from build123d import *

# Parameters (mm, degrees)
ESQUISSE1_W             = 8.5
ESQUISSE1_H             = 72
ESQUISSE1_R             = 2.1
BOSS_EXTRU_1_DEPTH      = 17.5
ENL_V_START             = -3
ENL_V_MAT_EXTRU_4_DEPTH = 3.5
ESQUISSE7_R             = 2.1
BOSS_EXTRU_3_DEPTH      = 8
ESQUISSE3_W             = 8.5
ESQUISSE3_H             = 4
ENL_V_MAT_EXTRU_3_DEPTH = 19
BOSS_EXTRU_2_START      = -7
BOSS_EXTRU_2_DEPTH      = 12
ESQUISSE8_W             = 8.5
ESQUISSE8_H             = 7
BOSS_EXTRU_4_DEPTH      = 4
ESQUISSE9_R             = 1.6
ENL_V_MAT_EXTRU_5_DEPTH = 5
ENL_V_START_2           = -4
ESQUISSE10_R            = 1.6
ENL_V_MAT_EXTRU_6_DEPTH = 2.6
ESQUISSE11_R            = 1.6
ENL_V_MAT_EXTRU_7_DEPTH = 1.6
ESQUISSE14_W            = 2.5
ESQUISSE14_H            = 10
ENL_V_MAT_EXTRU_9_DEPTH = 17.6
CHANFREIN1_SIZE         = 0.5


with BuildPart() as part:
    # Esquisse1 → Boss.-Extru.1 (new body)
    with BuildSketch(Plane.XY):
        with Locations((4.25, 36)):
            Rectangle(ESQUISSE1_W, ESQUISSE1_H)
        with Locations((4, 20.5)):
            Circle(ESQUISSE1_R, mode=Mode.SUBTRACT)
        with Locations((4, 51.5)):
            Circle(ESQUISSE1_R, mode=Mode.SUBTRACT)
    extrude(amount=BOSS_EXTRU_1_DEPTH)

    # Esquisse6 → Enlèv. mat.-Extru.4 (cut)
    with BuildSketch(Plane.XY.offset(17.5).offset(ENL_V_START)):
        Polygon((7.6, 22.578460969), (4, 24.656921938), (0.4, 22.578460969), (0.4, 18.421539031), (4, 16.343078062), (7.6, 18.421539031), align=None)
        Polygon((8.5, 24.656921938), (4, 24.656921938), (7.6, 22.578460969), (7.6, 18.421539031), (4, 16.343078062), (8.5, 16.343078062), align=None)
    enl_v_mat_extru_4 = extrude(amount=-ENL_V_MAT_EXTRU_4_DEPTH, mode=Mode.SUBTRACT)

    # Esquisse7 → Boss.-Extru.3 (add)
    with BuildSketch(Plane(origin=(0, 0, 0), x_dir=(-1, 0, 0), z_dir=(0, 0, -1))):
        with Locations((-4, 20.5)):
            Circle(ESQUISSE7_R)
    boss_extru_3 = extrude(amount=-BOSS_EXTRU_3_DEPTH)

    # Esquisse3 → Enlèv. mat.-Extru.3 (cut)
    with BuildSketch(Plane(origin=(0, 0, 0), x_dir=(-1, 0, 0), z_dir=(0, -1, 0))):
        with Locations((-4.25, -2)):
            Rectangle(ESQUISSE3_W, ESQUISSE3_H)
    enl_v_mat_extru_3 = extrude(amount=-ENL_V_MAT_EXTRU_3_DEPTH, mode=Mode.SUBTRACT)

    # Esquisse5 → Boss.-Extru.2 (add)
    with BuildSketch(Plane.XZ.offset(BOSS_EXTRU_2_START)):
        with BuildLine():
            ThreePointArc((4.662966643, 2.165487935), (4.682946936, 2.27184931), (4.714353535, 2.375413685))
            ThreePointArc((4.714353535, 2.375413685), (5.229781903, 2.78475984), (5.773646598, 2.414028307))
            ThreePointArc((5.773646598, 2.414028307), (5.814751932, 2.291920009), (5.839789089, 2.165534781))
            ThreePointArc((5.839789089, 2.165534781), (5.889607538, 2.072347427), (5.988503907, 2.035128225))
            Line((5.988503907, 2.035128225), (6.514258005, 2.035128225))
            ThreePointArc((6.514258005, 2.035128225), (6.613136609, 2.072331852), (6.662966643, 2.165487935))
            ThreePointArc((6.662966643, 2.165487935), (6.682946936, 2.27184931), (6.714353535, 2.375413685))
            ThreePointArc((6.714353535, 2.375413685), (7.229781903, 2.78475984), (7.773646598, 2.414028307))
            ThreePointArc((7.773646598, 2.414028307), (7.814751932, 2.291920009), (7.839789089, 2.165534781))
            ThreePointArc((7.839789089, 2.165534781), (7.889607538, 2.072347427), (7.988503907, 2.035128225))
            Line((7.988503907, 2.035128225), (8.5, 2.035128225))
            Line((8.5, 2.035128225), (8.5, 4))
            Line((8.5, 4), (0, 4))
            Line((0, 4), (0, 2.035128225))
            Line((0, 2.035128225), (0.514258005, 2.035128225))
            ThreePointArc((0.514258005, 2.035128225), (0.61313661, 2.072331853), (0.662966644, 2.165487937))
            ThreePointArc((0.662966644, 2.165487937), (0.682946936, 2.271849312), (0.714353535, 2.375413685))
            ThreePointArc((0.714353535, 2.375413685), (1.229781903, 2.78475984), (1.773646598, 2.414028307))
            ThreePointArc((1.773646598, 2.414028307), (1.814751932, 2.291920009), (1.839789089, 2.165534781))
            ThreePointArc((1.839789089, 2.165534781), (1.889607538, 2.072347427), (1.988503907, 2.035128225))
            Line((1.988503907, 2.035128225), (2.514258006, 2.035128225))
            ThreePointArc((2.514258006, 2.035128225), (2.613136611, 2.072331854), (2.662966644, 2.16548794))
            ThreePointArc((2.662966644, 2.16548794), (2.682946936, 2.271849313), (2.714353535, 2.375413685))
            ThreePointArc((2.714353535, 2.375413685), (3.229781903, 2.78475984), (3.773646598, 2.414028307))
            ThreePointArc((3.773646598, 2.414028307), (3.814751932, 2.291920009), (3.839789089, 2.165534781))
            ThreePointArc((3.839789089, 2.165534781), (3.889607538, 2.072347427), (3.988503907, 2.035128225))
            Line((3.988503907, 2.035128225), (4.514258005, 2.035128225))
            ThreePointArc((4.514258005, 2.035128225), (4.613136609, 2.072331852), (4.662966643, 2.165487935))
        make_face()
    boss_extru_2 = extrude(amount=-BOSS_EXTRU_2_DEPTH)

    # Esquisse8 → Boss.-Extru.4 (add)
    with BuildSketch(Plane(origin=(0, 0, 4), x_dir=(-1, 0, 0), z_dir=(0, 0, -1))):
        with Locations((-4.25, 3.5)):
            Rectangle(ESQUISSE8_W, ESQUISSE8_H)
    boss_extru_4 = extrude(amount=BOSS_EXTRU_4_DEPTH)

    # Esquisse9 → Enlèv. mat.-Extru.5 (cut)
    with BuildSketch(Plane(origin=(0, 0, 0), x_dir=(-1, 0, 0), z_dir=(0, 0, -1))):
        with Locations((-4.25, 3.75)):
            Circle(ESQUISSE9_R)
        with Locations((-4.25, 22.25)):
            Circle(ESQUISSE9_R)
    enl_v_mat_extru_5 = extrude(amount=-ENL_V_MAT_EXTRU_5_DEPTH, mode=Mode.SUBTRACT)

    # Esquisse10 → Enlèv. mat.-Extru.6 (cut)
    # profile 1 of 4: a face of its own
    with BuildSketch(Plane(origin=(0, 0, 0), x_dir=(-1, 0, 0), z_dir=(0, 0, -1)).offset(ENL_V_START_2)):
        Polygon((-2.604551733, 25.1), (-5.895448267, 25.1), (-7.540896534, 22.25), (-5.895448267, 19.4), (-2.604551733, 19.4), (-0.959103466, 22.25), align=None)
        with Locations((-4.25, 22.25)):
            Circle(ESQUISSE10_R, mode=Mode.SUBTRACT)
    # profile 2 of 4: a face of its own
    with BuildSketch(Plane(origin=(0, 0, 0), x_dir=(-1, 0, 0), z_dir=(0, 0, -1)).offset(ENL_V_START_2)):
        Polygon((-2.604551733, 6.6), (-5.895448267, 6.6), (-7.540896534, 3.75), (-5.895448267, 0.9), (-2.604551733, 0.9), (-0.959103466, 3.75), align=None)
    # profile 3 of 4: a face of its own
    with BuildSketch(Plane(origin=(0, 0, 0), x_dir=(-1, 0, 0), z_dir=(0, 0, -1)).offset(ENL_V_START_2)):
        Polygon((-8.5, 6.6), (-5.895448267, 6.6), (-7.540896534, 3.75), (-5.895448267, 0.9), (-8.5, 0.9), align=None)
    # profile 4 of 4: a face of its own
    with BuildSketch(Plane(origin=(0, 0, 0), x_dir=(-1, 0, 0), z_dir=(0, 0, -1)).offset(ENL_V_START_2)):
        Polygon((-7.540896534, 22.25), (-5.895448267, 25.1), (-8.5, 25.1), (-8.5, 19.4), (-5.895448267, 19.4), align=None)
    enl_v_mat_extru_6 = extrude(amount=-ENL_V_MAT_EXTRU_6_DEPTH, mode=Mode.SUBTRACT)

    # Esquisse11 → Enlèv. mat.-Extru.7 (cut)
    with BuildSketch(Plane(origin=(0, 0, 5), x_dir=(-1, 0, 0), z_dir=(0, 0, -1))):
        with Locations((-4.25, 22.25)):
            Circle(ESQUISSE11_R)
    enl_v_mat_extru_7 = extrude(amount=-ENL_V_MAT_EXTRU_7_DEPTH, mode=Mode.SUBTRACT)

    # Esquisse14 → Enlèv. mat.-Extru.9 (cut)
    with BuildSketch(Plane(origin=(8.5, 0, 0), x_dir=(0, 0, -1), z_dir=(1, 0, 0))):
        with Locations((-6.75, 13)):
            Rectangle(ESQUISSE14_W, ESQUISSE14_H)
    enl_v_mat_extru_9 = extrude(amount=-ENL_V_MAT_EXTRU_9_DEPTH, mode=Mode.SUBTRACT)

    # Symétrie14: Enlèv. mat.-Extru.4, Boss.-Extru.3, Enlèv. mat.-Extru.3, Boss.-Extru.2, Boss.-Extru.4, Enlèv. mat.-Extru.5, Enlèv. mat.-Extru.6, Enlèv. mat.-Extru.7, Enlèv. mat.-Extru.9 across plane
    add(enl_v_mat_extru_4.mirror(Plane(origin=(0, 36, 0), x_dir=(0, 0, 1), z_dir=(0, -1, 0))), mode=Mode.SUBTRACT)
    add(boss_extru_3.mirror(Plane(origin=(0, 36, 0), x_dir=(0, 0, 1), z_dir=(0, -1, 0))))
    add(enl_v_mat_extru_3.mirror(Plane(origin=(0, 36, 0), x_dir=(0, 0, 1), z_dir=(0, -1, 0))), mode=Mode.SUBTRACT)
    add(boss_extru_2.mirror(Plane(origin=(0, 36, 0), x_dir=(0, 0, 1), z_dir=(0, -1, 0))))
    add(boss_extru_4.mirror(Plane(origin=(0, 36, 0), x_dir=(0, 0, 1), z_dir=(0, -1, 0))))
    add(enl_v_mat_extru_5.mirror(Plane(origin=(0, 36, 0), x_dir=(0, 0, 1), z_dir=(0, -1, 0))), mode=Mode.SUBTRACT)
    add(enl_v_mat_extru_6.mirror(Plane(origin=(0, 36, 0), x_dir=(0, 0, 1), z_dir=(0, -1, 0))), mode=Mode.SUBTRACT)
    add(enl_v_mat_extru_7.mirror(Plane(origin=(0, 36, 0), x_dir=(0, 0, 1), z_dir=(0, -1, 0))), mode=Mode.SUBTRACT)
    add(enl_v_mat_extru_9.mirror(Plane(origin=(0, 36, 0), x_dir=(0, 0, 1), z_dir=(0, -1, 0))), mode=Mode.SUBTRACT)

    # Chanfrein1
    chanfrein1_edges = [part.edges().sort_by_distance(p)[0] for p in [
        (1.9, 51.5, 14.5),
        (1.9, 51.5, 11),
        (1.9, 20.5, 11),
        (1.9, 20.5, 14.5),
    ]]
    chamfer(chanfrein1_edges, length=CHANFREIN1_SIZE)


solid = part.part
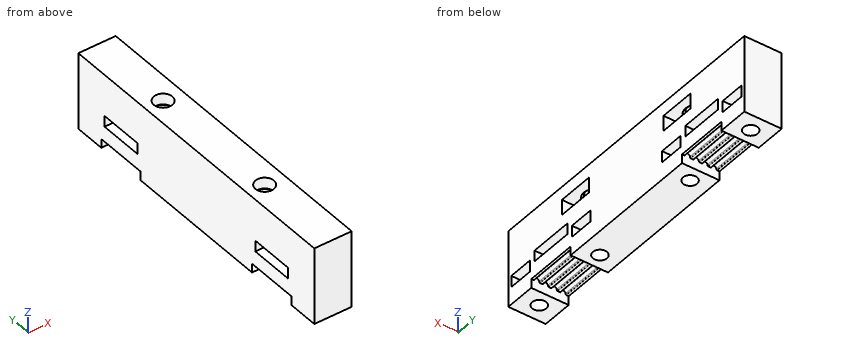
Part model, mm, in its own coordinate system. Give positions to 0.01 mm unless a question says otherwise; leave off trailing zeros. Order: outer loops, then holes, each group sorted by start corner. A loop starts at its lowest first (then second) coordinate and runs counter-clockwise, first axis right, second up. Notation, with made-up numbers: (54.5, 67) - (74.5, 67) arc R8 ccw to (74.5, 77) - close; hole circle Ø8 at (50.25, 13.25). An arc over 180 degrees is marked (long way). Use a Markdown table: item, result.
1) Flat gauge pin, fed straight in: P1, Ø4, axis at x = 5, y = 59, coming from the -Z side. Where does the tip first touch, or does it go through?
Checked values:
| item | result |
|---|---|
| P1 | z = 2.04 |
2) Probe L1, parallel to Y at x = 8, z = 5.25; L2, parallel to Z at x = 3.25, y = 47.5; L3, parallel to Z at x = 7.25, y = 49. List the from-to ranges inside material, lowest first. Write a range as from..to.
Checked values:
| item | result |
|---|---|
| L1 | 0..0.9, 6.6..19.4, 25.1..46.9, 52.6..65.4, 71.1..72 |
| L2 | 0..4, 6.6..17.5 |
| L3 | 0..4, 6.6..11, 14.5..17.5 |
3) Saw through at A-A on z = 13.25. List the corners of the cut face in (x, y).
Checked values:
| item | result |
|---|---|
| outline | (0, 0) - (8.5, 0) - (8.5, 16.34) - (4, 16.34) - (0.4, 18.42) - (0.4, 22.58) - (4, 24.66) - (8.5, 24.66) - (8.5, 47.34) - (4, 47.34) - (0.4, 49.42) - (0.4, 53.58) - (4, 55.66) - (8.5, 55.66) - (8.5, 72) - (0, 72) - close |
